Here's how the part is built. I have some questions about the finished solid (model axes, mm). A direction names the side the tool comes from. Round coordinates to 2 decimals unless told otherwise and drop trailing zeros. Write each loop counter-clockwise with the first axis right and the second up, starting at its lowest first coordinate (ties: lowest second). Pieces come first, ordered by that corner, then holes. Notation, with made-up numbers: (-25.5, -32) -> (-19.5, -32) arc R23 ccw to (-19.5, -15) -> close; hole circle Ø8 at (2.25, -11.5). An arc over 180 degrees is marked (long way). Put each result on its own line as item: value. Start each with the question number.
1) We'd pull the mould along X, two halves only. Please class faces 4 (the cylindrical face through (-19.5, -0.2, 0)), 5 (the cylindrical face through (-27.5, 0.1, 6.6)), 6 (the flat face through (-28, 0, -2.5)): released by +X, released by -X, zero draft, split by the parting line, or undercut.
2) Which directions (+Z, -Z, +X, -X, +Y, -Y) give clear straight access to the entire face, cutting with the end or side of a thin tool? Please do faces 1 (the flat face through (0, 6.2, -9.3)), 2 (the cylindrical face through (173.52, -2.17, -9.76)), 3 (the flat face through (-28, 0, 10.5)).
3) I want a section at C-C, the plane y = 0. Give the number of separate pieces and of enclosed holes in the cut face, then the cut area to 3 significant figures.
4) I want a section at A-A, the plane z = 0. List the corners of the cut face in (x, y) for me, then the cut area to 3 significant figures.
5) Will these pins go through, and if not, where does the flat tip stop? P1, Ø3, axis at x = 75, z = 6, coming from the +Y side; P2, Ø7, axis at y = -6, z = -4.5, coming from the -X side; P3, Ø6, axis at x = -25.5, y = -1, coming from the -Z side.
6) I want a section at B-B, the plane x = 86.5. List the corners of the cut face in (y, z) for me, then the cut area to 3 significant figures.
7) If I drill on line 1 along Z through (x, y) = (45, 0.5); line 2 along Z through (x, y) = (-28, -3.25); line 3 along X through (y, z) = (12.5, 2.25), over which ranges is the centre line in solid material (lowest first)? Write a range as [from, to].
from build123d import *

# Parameters (mm, degrees)
SKETCH6_OUTSIDE_W       = 75.24
SKETCH6_OUTSIDE_H       = 75.24
SKETCH6_OUTSIDE_W_2     = 21
SKETCH6_OUTSIDE_H_2     = 30
CUT_EXTRUDE3_DEPTH      = 40
SKETCH4_W               = 17.5
SKETCH4_H               = 5
FILLET1_R               = 1
SKETCH8_R               = 2.5
CUT_EXTRUDE4_DEPTH      = 5.5
CUT_EXTRUDE4_DEPTH_BACK = 26.5


with BuildPart() as part:
    # Sketch1 → Revolve1 (revolve)
    with BuildSketch(Plane.XY):
        with BuildLine():
            Line((172, 10), (175, 10))
            Line((175, 10), (175, 15))
            Line((175, 15), (0, 15))
            Line((0, 15), (0, 10))
            Line((0, 10), (-18.366750419, 10))
            ThreePointArc((-18.366750419, 10), (-30.674548662, 10.573528147), (-37, 0))
            Line((-37, 0), (0, 0))
            Line((0, 0), (3, 0))
            Line((3, 0), (3, 12))
            Line((3, 12), (172, 12))
            Line((172, 12), (172, 10))
        make_face()
    revolve(axis=Axis((0, 0, 0), (1, 0, 0)))

    # Sketch6 outside → Cut-Extrude3 (cut)
    with BuildSketch(Plane.ZY):
        Rectangle(SKETCH6_OUTSIDE_W, SKETCH6_OUTSIDE_H)
        Rectangle(SKETCH6_OUTSIDE_W_2, SKETCH6_OUTSIDE_H_2, mode=Mode.SUBTRACT)
    extrude(amount=CUT_EXTRUDE3_DEPTH, mode=Mode.SUBTRACT)

    # Sketch4 → Cut-Revolve1 (revolve, cut)
    with BuildSketch(Plane(origin=(0, 0, 0), x_dir=(1, 0, 0), z_dir=(0, 1, 0))):
        with Locations((-28.25, 0)):
            Rectangle(SKETCH4_W, SKETCH4_H)
    revolve(axis=Axis((-37, 0, -2.5), (0, 0, 1)), mode=Mode.SUBTRACT)

    # Fillet1
    fillet1_edges = [part.edges().sort_by_distance(p)[0] for p in [
        (175, -15, 0),
        (0, -15, 0),
        (0, -10, 0),
        (0, -15, 0),
    ]]
    fillet(fillet1_edges, radius=FILLET1_R)

    # Sketch8 → Cut-Extrude4 (cut, two sides)
    with BuildSketch(Plane.XY.offset(10.5)) as cut_extrude4_sk:
        with Locations((-25, 0)):
            Circle(SKETCH8_R)
    extrude(amount=CUT_EXTRUDE4_DEPTH, mode=Mode.SUBTRACT)
    extrude(cut_extrude4_sk.sketch, amount=-CUT_EXTRUDE4_DEPTH_BACK, mode=Mode.SUBTRACT)


solid = part.part
Findings:
1. face 4: released by -X
1. face 5: undercut
1. face 6: zero draft
2. face 1: none
2. face 2: +X
2. face 3: +Z, -X, +Y, -Y
3. separate pieces: 3
3. enclosed holes: 0
3. area: 1,690 mm2
4. outline: (-24.24, -11.98) arc R12 ccw to (-18.37, -10) -> (-1, -10) arc R1 cw to (0, -11) -> (0, -14) arc R1 ccw to (1, -15) -> (174, -15) arc R1 ccw to (175, -14) -> (175, -10) -> (172, -10) -> (172, -12) -> (3, -12) -> (3, 12) -> (172, 12) -> (172, 10) -> (175, 10) -> (175, 14) arc R1 ccw to (174, 15) -> (1, 15) arc R1 ccw to (0, 14) -> (0, 11) arc R1 cw to (-1, 10) -> (-18.37, 10) arc R12 ccw to (-24.24, 11.98) arc R17.5 cw to start
4. area: 1,560 mm2
5. P1: stops at y = 14.31
5. P2: stops at x = -36.31
5. P3: stops at z = -10.5
6. outline: circle Ø30 at (0, 0); hole circle Ø24 at (0, 0)
6. area: 254 mm2
7. line 1: z = [-14.99, -11.99], [11.99, 14.99]
7. line 2: z = [-10.5, -2.5], [2.5, 10.5]
7. line 3: x = [0, 175]
